```python
from build123d import *

# Parameters (mm, degrees)
SKETCH1_R           = 20
SKETCH1_R_2         = 4
BOSS_EXTRUDE1_DEPTH = 10
CUT_EXTRUDE1_DEPTH  = 7
SKETCH4_R           = 2.125
CUT_EXTRUDE2_DEPTH  = 3.000006


with BuildPart() as part:
    # Sketch1 → Boss-Extrude1 (new body)
    with BuildSketch(Plane(origin=(0, 0, 0), x_dir=(1, 0, 0), z_dir=(0, 1, 0))):
        Circle(SKETCH1_R)
        Circle(SKETCH1_R_2, mode=Mode.SUBTRACT)
    extrude(amount=BOSS_EXTRUDE1_DEPTH)

    # Sketch3 → Cut-Extrude1 (cut)
    with BuildSketch(Plane(origin=(0, 0, 0), x_dir=(1, 0, 0), z_dir=(0, 1, 0))):
        with BuildLine():
            Line((-12.000006, 3.320491078), (-12.000006, -3.320491078))
            ThreePointArc((-12.000006, -3.320491078), (-15, -4.475), (-17.999994, -3.320491078))
            Line((-17.999994, -3.320491078), (-17.999994, 3.320491078))
            ThreePointArc((-17.999994, 3.320491078), (-15, 4.475), (-12.000006, 3.320491078))
        make_face()
    extrude(amount=CUT_EXTRUDE1_DEPTH, mode=Mode.SUBTRACT)

    # Sketch4 → Cut-Extrude2 (cut, through all)
    with BuildSketch(Plane(origin=(-17.999994, 0, 0), x_dir=(0, 0, -1), z_dir=(1, 0, 0))):
        with Locations((0, 3)):
            Circle(SKETCH4_R)
    extrude(amount=-CUT_EXTRUDE2_DEPTH, mode=Mode.SUBTRACT)


solid = part.part
```
CAD build for the part. Positions are in the model's coordinates, mm. A direction names the side the tool comes from. Give positions to 0.01 mm unless a question says otherwise; leave off trailing zeros. Write each loop counter-clockwise with the first axis right and the second up, starting at its lowest first coordinate (ties: lowest second). Pieces come first, ordered by that corner, then holes. Notation, with made-up numbers: M 44,1.5 L 85,1.5 A26 ccw 85,29.5 Z; hole C -35,-30 d10. An arc over 180 degrees is marked long. Return JSON: item names as keys, results as strings. Group by question number.
(1) Band-saw the part on B-B (z = 0). Give the cut face in (x, y) (3 decimals), and give its area (4 significant figures).
(2) Flat gauge pins, fed straight in: pin 1 Ø5 at (y, z) = (1.5, -7.5) entering from -X; pin 2 Ø2 at (y, z) = (4.5, 15) entering from +X; pin 3 Ø3 at (x, z) = (-15, -0.5) entering from -Y. Where does each tip first touch, or does it go through?
(3) Drill centre lines: L1, parallel to Z at x = 0, y = 6.25; L2, parallel to X at y = 4.25, z = 0; L3, parallel to X at y = 0.5, z = 2. Where is each one in solid material? Low to high. Write a range as [from, to].
(4) 3-axis set-ups, long thin cutter, end or side, ignore diameter. For faces 4 (the face through (-12, 3, 0)), 5 (the face through (-18.986, 0.926, 0.461)), 6 (the face through (4.2, 10, -0.3)): which of +Z, -Z, +X, -X, +Y, -Y reach the whole face in a straight line?
(5) Band-saw the part on A-A (x = 0). Give the cut face in (y, z).
(6) Mould opens along X. For faces 1 (the face through (4.2, 0, -0.3)), 2 (the face through (19.076, 4.93, -6.007)), 3 (the face through (-14.954, 3.451, 4.475)) say: pulls with the +X half, pulls with the -X half, needs draft (parallel to the pull), parting line crosses it, or undercut.
(7) Band-saw the part on D-D (x = -15.5). Give the cut face in (y, z), and give its area (3 significant figures).
Entries:
{
 "1": {"outline": "M -20,0 L -18,0 L -18,0.875 L -20,0.875 Z; M -20,5.125 L -18,5.125 L -18,7 L -12,7 L -12,0 L -4,0 L -4,10 L -20,10 Z; M 4,0 L 20,0 L 20,10 L 4,10 Z", "area": "269.5 mm^2"},
 "2": {"pin 1": "stops at x = -19.36", "pin 2": "stops at x = 14.28", "pin 3": "stops at y = 7"},
 "3": {"L1": "z = [-20, -4], [4, 20]", "L2": "x = [-12, -4], [4, 20]", "L3": "x = [-19.9, -18], [-12, -3.46], [3.46, 19.9]"},
 "4": {"face 4": "-Y", "face 5": "-X", "face 6": "+Z, -Z, +X, -X, +Y"},
 "5": {"outline": "M 0,-20 L 10,-20 L 10,-4 L 0,-4 Z; M 0,4 L 10,4 L 10,20 L 0,20 Z"},
 "6": {"face 1": "needs draft", "face 2": "parting line crosses it", "face 3": "undercut"},
 "7": {"outline": "M 0,-12.64 L 10,-12.64 L 10,12.64 L 0,12.64 L 0,4.45 L 7,4.45 L 7,-4.45 L 0,-4.45 Z", "area": "191 mm^2"}
}
